from build123d import *

# Parameters (mm, degrees)
F1_DEPTH = 3


with BuildPart() as f1:
    # F0 (on Front) → F1 (new body)
    with BuildSketch(Plane.XZ):
        with BuildLine():
            Line((-14.696938, 41.45), (-10, 41.45))
            Line((-10, 41.45), (-10, 0))
            ThreePointArc((-10, 0), (-7.582875, -6.519202), (-1.5, -9.88686))
            Line((-1.5, -9.88686), (-1.5, 15))
            Line((-1.5, 15), (1.5, 15))
            Line((1.5, 15), (1.5, -9.88686))
            ThreePointArc((1.5, -9.88686), (7.582875, -6.519202), (10, 0))
            Line((10, 0), (10, 41.45))
            Line((10, 41.45), (14.696938, 41.45))
            ThreePointArc((14.696938, 41.45), (0, 53.45), (-14.696938, 41.45))
        make_face()
    extrude(amount=F1_DEPTH)


solid = f1.part
Input: part model. Units: mm. Frame: model coordinates. A direction names the side the tool comes from. Coordinates: 2 decimals unless noted, no trailing zeros. Loops run counter-clockwise (first coordinate to the right, second up) from the corner with the lowest first, then second, coordinate; pieces in that order, holes last.
Q1. Cut plane B-B (y = -0.6). Output: boundary loops of the cut face in (x, z).
Q2. Draft query along X for faces 1 (the face through (10, -1, 20)), 2 (the face through (0, -3, 22)), 3 (the face through (0, -1, 15)), 4 (the face through (0.288, -1.479, 53.447)). Return one class per face: +X half, -X half, draft (parallel to the pull), parting line (faces both ways), or undercut.
Q3. Cut plane D-D (z = 37.5). Output: boundary loops of the cut face in (x, y), then the cut area to 3 significant figures.
Q4. Set-up query: faces 5 (the face through (12, -1, 41.45)), 6 (the face through (0, 0, 22)), 7 (the face through (-12, -1, 41.45)), 8 (the face through (-1.5, -1, 2)). Return all of +Z, -Z, +X, -X, +Y, -Y with unobstructed straight access to the full face (end or side cutting, diameter ignored); none if empty.
Q5. Contact query for flat-ended pins moving along their axis: pin 1 (0.9 mm diameter, centred on y = -1, z = 7, fed in from +X); pin 2 (1.5 mm diameter, centred on x = -12, y = -2, fed in from -Z); pin 3 (4 mm diameter, centred on x = -0.5, z = -2.5, fed in from -Y); pin 4 (1 mm diameter, centred on x = -3.5, y = -0.5, fed in from -Z). Output: stop coordinate, or through.
Q6. Material intervals for line 1 (X direction, y = -1, z = 12); line 2 (X direction, y = -2.45, z = 21); line 3 (X direction, y = -1.45, z = -1.5), sorted ascending.
Q7. Cut plane A-A (z = 9). Output: boundary loops of the cut face in (x, y), then the cut area to 3 significant figures.
Q8. Cut plane C-C (x = 12). Output: boundary loops of the cut face in (y, z).
Working result:
1. outline: (-14.7, 41.45) - (-10, 41.45) - (-10, 0) arc R10 ccw to (-1.5, -9.89) - (-1.5, 15) - (1.5, 15) - (1.5, -9.89) arc R10 ccw to (10, 0) - (10, 41.45) - (14.7, 41.45) arc R15 ccw to start
2. face 1: +X half
2. face 2: draft
2. face 3: undercut
2. face 4: parting line
3. outline: (-10, -3) - (10, -3) - (10, 0) - (-10, 0) - close
3. area: 60.0 mm2
4. face 5: -Z, +X, +Y, -Y
4. face 6: +Z, -Z, +X, -X, +Y
4. face 7: -Z, -X, +Y, -Y
4. face 8: -Z, +Y, -Y
5. pin 1: stops at x = 10
5. pin 2: stops at z = 41.45
5. pin 3: stops at y = -3
5. pin 4: stops at z = -9.54
6. line 1: x = -10 to -1.5, 1.5 to 10
6. line 2: x = -10 to 10
6. line 3: x = -9.89 to -1.5, 1.5 to 9.89
7. outline: (-10, -3) - (-1.5, -3) - (-1.5, 0) - (-10, 0) - close; (1.5, -3) - (10, -3) - (10, 0) - (1.5, 0) - close
7. area: 51.0 mm2
8. outline: (-3, 41.45) - (0, 41.45) - (0, 47.45) - (-3, 47.45) - close
